Geometry: final body of the model. Coordinates: model frame, mm. A direction names the side the tool comes from. Give positions to 0.01 mm unless a question says otherwise; leave off trailing zeros. Loops run counter-clockwise (first coordinate to the right, second up) from the corner with the lowest first, then second, coordinate; pieces in that order, holes last. Notation, with made-up numbers: (77.5, 4.25) - (123.5, 4.25) arc R21 ccw to (123.5, 14.25) - close; hole circle Ø3 at (41.25, 73). An arc over 180 degrees is marked (long way). Answer in a Markdown table with one row per item.
from build123d import *

# Parameters (mm, degrees)
F1_DEPTH = 152.4
F3_R     = 12.7
F4_DEPTH = 25.4
F5_R     = 12.7
F6_DEPTH = 25.4


# Not quite as in the source:
# - a pattern or mirror of a feature is missing from the dataset's text; its kind, count and spacing are read off the source's solid


with BuildPart() as f1:
    # F0 (on Right) → F1 (new body)
    with BuildSketch(Plane.YZ):
        with BuildLine():
            Line((63.5, 12.7), (63.5, 76.2))
            ThreePointArc((63.5, 76.2), (0, 139.7), (-63.5, 76.2))
            Line((-63.5, 76.2), (-63.5, 12.7))
            Line((-63.5, 12.7), (-63.5, 0))
            Line((-63.5, 0), (63.5, 0))
            Line((63.5, 0), (63.5, 12.7))
        make_face()
    extrude(amount=-F1_DEPTH)

    # F3 (on Top) → F4 (join)
    with BuildSketch(Plane.XY):
        with BuildLine():
            Line((0, 90.7872649688), (-0.002730534, 90.7872649688))
            ThreePointArc((-0.002730534, 90.7872649688), (-25.401365267, 115.9239140637), (-50.8, 90.7872649688))
            Line((-50.8, 90.7872649688), (-50.8, 63.5))
            Line((-50.8, 63.5), (0, 63.5))
            Line((0, 63.5), (0, 90.7872649688))
        make_face()
        with Locations((-25.401365267, 90.5239140637)):
            Circle(F3_R, mode=Mode.SUBTRACT)
        with BuildLine():
            Line((-101.6, 90.7872649688), (-101.602730534, 90.7872649688))
            ThreePointArc((-101.602730534, 90.7872649688), (-127.001365267, 115.9239140637), (-152.4, 90.7872649688))
            Line((-152.4, 90.7872649688), (-152.4, 63.5))
            Line((-152.4, 63.5), (-101.6, 63.5))
            Line((-101.6, 63.5), (-101.6, 90.7872649688))
        make_face()
        with Locations((-127.001365267, 90.5239140637)):
            Circle(F3_R, mode=Mode.SUBTRACT)
    f4 = extrude(amount=F4_DEPTH)

    # F4_copies: F4 across plane
    add(f4.mirror(Plane(origin=(0, 0, 0), x_dir=(0, 0, -1), z_dir=(0, -1, 0))))

    # F5 (on face) → F6 (cut)
    with BuildSketch(Plane.YZ):
        with Locations((0, 76.3214752078)):
            Circle(F5_R)
    extrude(amount=-F6_DEPTH, mode=Mode.SUBTRACT)


solid = f1.part
Q1. Cut plane D-D (z = 19). Give the number of separate pieces and of enclosed holes in the cut face, and give its area (3 significant figures).
Check values:
| item | result |
|---|---|
| separate pieces | 1 |
| enclosed holes | 4 |
| area | 26,900 mm² |
Q2. Material intervals for line 1 along X through (y, z) = (100, 21); line 2 along X through (y, z) = (-81, 22.5); line 3 along Y through (x, z) = (-86.5, 18.5), sorted ascending.
Check values:
| item | result |
|---|---|
| line 1 | -150.57 to -135.46, -118.55 to -103.44, -48.97 to -33.86, -16.95 to -1.84 |
| line 2 | -152.4 to -135.4, -118.6 to -101.6, -50.8 to -33.8, -17 to 0 |
| line 3 | -63.5 to 63.5 |
Q3. Draft query along Y for faces 1 (the flat face through (-50.8, 77, 13)), 2 (the cylindrical face through (-27.055, 103.116, 12.522)), 3 (the cylindrical face through (-24.847, 115.918, 12.522)). Return one class per face: pulls with the +Y half, pulls with the -Y half, needs draft (parallel to the pull), parting line crosses it, or undercut.
Check values:
| item | result |
|---|---|
| face 1 | needs draft |
| face 2 | undercut |
| face 3 | pulls with the +Y half |
Q4. First-contact query: pin 1 (15 mm diameter, centred on x = -23.5, y = 78.5, fed in from +Z); pin 2 (6 mm diameter, centred on x = -28.5, z = 103.5, fed in from +Y); pin 3 (8 mm diameter, centred on x = -29.5, z = 82, fed in from +Y); pin 4 (23 mm diameter, centred on x = -127, y = -90.52, fed in from -Z). Flat tips, straight axial feed; report the tip coordinate or a pass-through.
Check values:
| item | result |
|---|---|
| pin 1 | z = 25.4 |
| pin 2 | y = 58.67 |
| pin 3 | y = 63.47 |
| pin 4 | through |
Q5. Reachability of faces 4 (the flat face through (-101.6, 77, 13)), 5 (the cylindrical face through (-12.522, -1.653, 88.913)), 6 (the flat face through (-122, 78, 25.4)), 7 (the flat face through (-50.8, -77, 13)) from +Z, -Z, +X, -X, +Y, -Y: full face, straight path, thin tool, end or side. Return the list, or none.
Check values:
| item | result |
|---|---|
| face 4 | +Z, -Z, +Y |
| face 5 | +X |
| face 6 | +Z, +X, -X, +Y |
| face 7 | +Z, -Z, -Y |
Q6. Cut plane A-A (x = -127). Output: boundary loops of the cut face in (y, z), and give its area (3 significant figures).
Check values:
| item | result |
|---|---|
| outline | (-115.92, 0) - (-103.22, 0) - (-103.22, 25.4) - (-115.92, 25.4) - close; (-77.82, 0) - (77.82, 0) - (77.82, 25.4) - (63.5, 25.4) - (63.5, 76.2) arc R63.5 ccw to (-63.5, 76.2) - (-63.5, 25.4) - (-77.82, 25.4) - close; (103.22, 0) - (115.92, 0) - (115.92, 25.4) - (103.22, 25.4) - close |
| area | 17,400 mm² |
Q7. Cut plane B-B (y = 0). Output: boundary loops of the cut face in (x, z), and give its area (3 significant figures).
Check values:
| item | result |
|---|---|
| outline | (-152.4, 0) - (0, 0) - (0, 63.62) - (-25.4, 63.62) - (-25.4, 89.02) - (0, 89.02) - (0, 139.7) - (-152.4, 139.7) - close |
| area | 20,600 mm² |
Q8. Cut plane C-C (y = 84). Output: boundary loops of the cut face in (x, z).
Check values:
| item | result |
|---|---|
| outline | (-152.4, 0) - (-137.9, 0) - (-137.9, 25.4) - (-152.4, 25.4) - close; (-116.11, 0) - (-101.6, 0) - (-101.6, 25.4) - (-116.11, 25.4) - close; (-50.8, 0) - (-36.3, 0) - (-36.3, 25.4) - (-50.8, 25.4) - close; (-14.51, 0) - (0, 0) - (0, 25.4) - (-14.51, 25.4) - close |
